For this review, take the finished solid that the model builds, in its own axes (mm). Face numbers are marked on the shaded views. A direction names the side the tool comes from. Give positions to 0.01 mm unless a question says otherwise; leave off trailing zeros. Order: outer loops, then holes, each group sorted by start corner. A loop starts at its lowest first (then second) coordinate and runs counter-clockwise, first axis right, second up. Notation, with made-up numbers: M 28,20 L 87,20 A22 cw 87,34 Z; hole C 34,64 d1. An arc over 180 degrees is marked long. Answer as CSV lines item,"result". Start each with the question number.
1. We need section C-C, the plane x = -0.65. Give the boundary of the cut face in (y, z).
2. Clearance check with flat-ended pins moving along their axes: P1, Ø2, axis at y = 9.5, z = 9, coming from the +X side; P2, Ø5.5, axis at x = -13, z = 7, coming from the -Y side; P3, Ø6, axis at x = -1, z = 5.5, coming from the +Y side; P4, Ø3, axis at x = -11.5, z = 1.5, coming from the +Y side. State where each tip first meets the part, or that it passes through.
3. For line 1 along Z through (x, y) = (13.9, 6.6); line 2 along Y through (x, z) = (9, 9.5); line 3 along Y through (x, z) = (-2, 9), list the stretches that pass through material, from the lowest coordinate up.
4. We need section D-D, the plane z = 11. Give the boundary of the cut face in (x, y), and give its area (3 significant figures).
5. We need section B-B, the plane y = 17.5. Give the boundary of the cut face in (x, z).
6. Machinability: for the marked faces 1, 2, 3 and 4, which of the approach directions +Z, -Z, +X, -X, +Y, -Y give a long, thin tool a straight path to every point of the face, cutting with its end or side? Answer none if there is none.
7. We need section A-A, the plane x = 13.9. Give the boundary of the cut face in (y, z), and give its area (3 significant figures).
Autodesk Fusion 360 part; units mm, degrees
sketch "Sketch1" plane through (0, 0, 0) normal (0, 0, 1) x (1, 0, 0)
  line L0 (11.5, -12.1) -> (-11.5, -12.1)
  line L1 (-11.5, 12.1) -> (11.5, 12.1)
  line L2 (11.5, -12.1) -> (-11.5, 12.1) construction
  line L3 (-11.5, -12.1) -> (11.5, 12.1) construction
  line L4 (11.5, 7.6) -> (16.3, 7.6)
  line L5 (16.3, 7.6) -> (16.3, 5.2)
  line L6 (16.3, 5.2) -> (11.5, 5.2)
  line L7 (-16.3, 5.2) -> (-11.5, 5.2)
  line L8 (-16.3, 7.6) -> (-16.3, 5.2)
  line L9 (-11.5, 7.6) -> (-16.3, 7.6)
  line L10 (11.5, 12.1) -> (11.5, 7.6)
  line L11 (11.5, 5.2) -> (11.5, -12.1)
  line L12 (-11.5, -12.1) -> (-11.5, 5.2)
  line L13 (-11.5, 7.6) -> (-11.5, 12.1)
  dimension "d1" = 23
  dimension "d2" = 24.2
  dimension "d3" = 4.5
  dimension "d4" = 4.8
  dimension "d5" = 2.4
extrude "Extrude1" add sketch "Sketch1" along normal blind 12.1
sketch "Sketch2" plane through (0, 7.6, 0) normal (0, 1, 0) x (-1, 0, 0)
  line L0 (-16.3, 0) -> (-11.5, 0)
  line L1 (-11.5, 0) -> (-11.5, 12.1)
  line L2 (-11.5, 12.1) -> (-16.3, 12.1)
  line L3 (-16.3, 12.1) -> (-16.3, 0)
  circle A0 centre (14, 6) radius 1.5
  circle A1 centre (-13.9, 6.05) radius 1.5
  dimension "d8" = 3
  dimension "d9" = 3
extrude "Extrude2" cut sketch "Sketch2" against normal blind 5 contours A0 | A1
sketch "Sketch3" plane through (0, 12.1, 0) normal (0, 1, 0) x (-1, 0, 0)
  line L0 (-11.5, 0) -> (11.5, 0)
  line L1 (11.5, 0) -> (11.5, 12.1)
  line L2 (11.5, 12.1) -> (-11.5, 12.1)
  line L3 (-11.5, 12.1) -> (-11.5, 0)
  line L4 (0.6, 6.05) -> (0.65, 6.05)
  arc A0 (0.0672, 3.5675) -> (0.0672, 8.5325) centre (0.65, 6.05) ccw
  arc A1 (0.0672, 8.5325) -> (0.0672, 3.5675) centre (-5.45, 6.05) ccw
  dimension "d12" = 6.1
  dimension "d13" = 5.1
extrude "Extrude3" add sketch "Sketch3" along normal blind 4.4 contours A0 A1
sketch "Sketch4" plane through (0, 16.5, 0) normal (0, 1, 0) x (-1, 0, 0)
  arc A0 (0.0672, 8.5325) -> (0.0672, 3.5675) centre (-5.45, 6.05) ccw
  arc A1 (0.0672, 3.5675) -> (0.0672, 8.5325) centre (0.65, 6.05) ccw
  circle A2 centre (-5.45, 6.05) radius 2.35
  line L0 (-4.4572, 3.92) -> (-3.5252, 4.7018)
  line L1 (-3.5252, 4.7018) -> (-3.109, 5.8448)
  line L2 (-3.109, 5.8448) -> (-3.32, 7.0428)
  line L3 (-3.32, 7.0428) -> (-4.1018, 7.9748)
  line L4 (-4.1018, 7.9748) -> (-5.2448, 8.391)
  line L5 (-5.2448, 8.391) -> (-6.4428, 8.18)
  line L6 (-6.4428, 8.18) -> (-7.3748, 7.3982)
  line L7 (-7.3748, 7.3982) -> (-7.791, 6.2552)
  line L8 (-7.791, 6.2552) -> (-7.58, 5.0572)
  line L9 (-7.58, 5.0572) -> (-6.7982, 4.1252)
  line L10 (-6.7982, 4.1252) -> (-5.6552, 3.709)
  line L11 (-5.6552, 3.709) -> (-4.4572, 3.92)
  point P0 (-5.45, 6.05)
  dimension "d16" = 4.7
extrude "Extrude4" add sketch "Sketch4" along normal blind 3.6 contours L0 L1 L2 L3 L4 L5 L6 L7 L8 L9 L10 L11
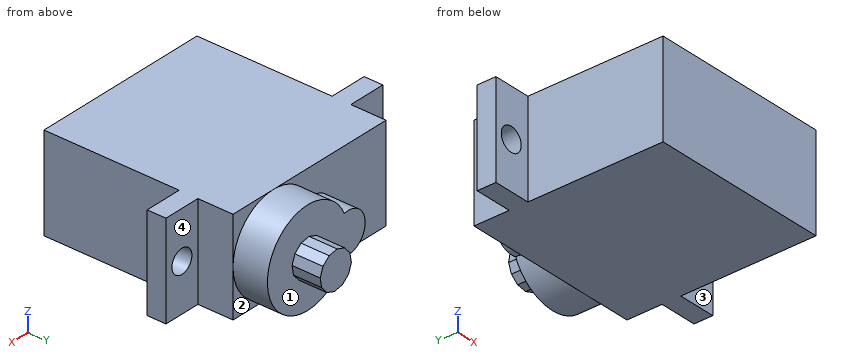
Result set:
1,outline,"M -12.1,0 L 12.1,0 L 12.1,3.5 L 16.5,3.5 L 16.5,8.6 L 12.1,8.6 L 12.1,12.1 L -12.1,12.1 Z"
2,P1,"x = 11.5"
2,P2,"y = -12.1"
2,P3,"y = 16.5"
2,P4,"y = 12.1"
3,line 1,"0 to 4.55, 7.55 to 12.1"
3,line 2,"-12.1 to 16.5"
3,line 3,"-12.1 to 12.1"
4,outline,"M -16.3,5.2 L -11.5,5.2 L -11.5,-12.1 L 11.5,-12.1 L 11.5,5.2 L 16.3,5.2 L 16.3,7.6 L 11.5,7.6 L 11.5,12.1 L 8.93,12.1 L 8.93,16.5 L 1.97,16.5 L 1.97,12.1 L -11.5,12.1 L -11.5,7.6 L -16.3,7.6 Z"
4,area,"610 mm2"
5,outline,"M 3.11,5.84 L 3.53,4.7 L 4.46,3.92 L 5.66,3.71 L 6.8,4.13 L 7.58,5.06 L 7.79,6.26 L 7.37,7.4 L 6.44,8.18 L 5.24,8.39 L 4.1,7.97 L 3.32,7.04 Z"
6,face 1,"+Y"
6,face 2,"-Z, +X, +Y"
6,face 3,"+Z, -Z, +X, -Y"
6,face 4,"+Z, -Z, +X, +Y"
7,outline,"M 5.2,0 L 7.6,0 L 7.6,4.55 L 5.2,4.55 Z; M 5.2,7.55 L 7.6,7.55 L 7.6,12.1 L 5.2,12.1 Z"
7,area,"21.8 mm2"
